The listing builds one solid part. Answer for the finished solid, in the listing's coordinates (mm). A direction names the side the tool comes from. Give positions to 0.01 mm unless a question says otherwise; leave off trailing zeros. Order: outer loops, then holes, each group sorted by start corner. A loop starts at its lowest first (then second) coordinate and runs counter-clockwise, first axis right, second up. Notation, with made-up numbers: (70.25, 67.5) - (93.25, 67.5) arc R31 ccw to (93.25, 106.5) - close; hole circle Ø4 at (-19, 72.5). An arc over 180 degrees is marked (long way). Use a Markdown table: item, result. Add a question column.
1) Flat-ended cylindrical pins translate along their axes: pin 1 (0.9 mm diameter, centred on x = 36, z = 3.5, fed in from +Y); pin 2 (3.5 mm diameter, centred on x = -31.5, z = 2.5, fed in from -Y); pin 3 (1.8 mm diameter, centred on x = 12.5, z = 2, fed in from -Y). Find the tip coordinate at first contact, or state that the pin passes through.
2) For faces 4 (the face through (-28.752, -19.875, 3.042)), 5 (the face through (11.39, -18.34, 2.96)), 6 (the face through (0, 11, 3)), 7 (the face through (38.483, 8.961, 3.042)), 8 (the face through (-8.11, 70.83, 3.04)), determine the directions among +Z, -Z, +X, -X, +Y, -Y from which every point of the face is accessible in a straight line to the end or side of a thin tool.
3) Find section B-B, the plane x = 13. Determine the outline of the cut face in (y, z), plus the area to 3 significant figures.
4) Find section C-C, the plane y = 47. Determine the outline of the cut face in (x, z).
5) Straight lines are drawn through the part: line 1 (X direction, y = 4.5, z = 0.4); line 2 (X direction, y = 11.5, z = 2.5); line 3 (X direction, y = 7.5, z = 0.85). For each, find the intervals that lie inside material, in ascending order.
6) Find section D-D, the plane x = -3.5. Determine the outline of the cut face in (y, z), plus the area to 3 significant figures.
7) The mould has two halves that part along X. Classify faces 1 (the face through (-28, 0, 3)), 2 (the face through (-18, 71.455, 3)), 3 (the face through (-27.851, 70.864, 3.042)): released by +X, released by -X, zero draft, split by the parting line, or undercut.
8) Find section A-A, the plane y = -11. Determine the outline of the cut face in (x, z).
from build123d import *

# Parameters (mm, degrees)
F1_DEPTH = 6
F2_R     = 2.5
F3_R     = 1.5


with BuildPart() as f1:
    # F0 (on Top) → F1 (new body)
    with BuildSketch(Plane.XY):
        with BuildLine():
            Line((30, 0), (0, 0))
            Line((0, 0), (0, 20))
            Line((0, 20), (-7.605883, 71.455397))
            Line((-7.605883, 71.455397), (-28.394117, 71.455397))
            Line((-28.394117, 71.455397), (-36, 20))
            Line((-36, 20), (-36, -20.588065))
            Line((-36, -20.588065), (-28, -20.588065))
            Line((-28, -20.588065), (-28, 19.411935))
            Line((-28, 19.411935), (-22, 60.003195))
            ThreePointArc((-22, 60.003195), (-18, 63.455397), (-14, 60.003195))
            Line((-14, 60.003195), (-8, 19.411935))
            Line((-8, 19.411935), (-8, -37))
            ThreePointArc((-8, -37), (-5.506746, -40.705363), (-1.135141, -39.79152))
            Line((-1.135141, -39.79152), (35.638156, -2.052121))
            Line((35.638156, -2.052121), (40.024769, 10))
            Line((40.024769, 10), (33.639702, 10))
            Line((33.639702, 10), (30, 0))
        make_face()
        Polygon((-1, -31.055363), (-1, -6), (23.413963, -6), align=None, mode=Mode.SUBTRACT)
    extrude(amount=F1_DEPTH)

    # F2
    f2_edges = [f1.edges().sort_by_distance(p)[0] for p in [
        (-36, 20, 3),
        (-28.394117, 71.455397, 3),
        (-7.605883, 71.455397, 3),
        (33.639702, 10, 3),
        (40.024769, 10, 3),
        (-8, 19.411935, 3),
        (0, 20, 3),
        (0, 0, 3),
        (30, 0, 3),
        (35.638156, -2.052121, 3),
        (-1, -6, 3),
        (-36, -20.588065, 3),
        (-28, -20.588065, 3),
        (-28, 19.411935, 3),
    ]]
    fillet(f2_edges, radius=F2_R)

    # F3
    f3_edges = [f1.edges().sort_by_distance(p)[0] for p in [
        (23.413963, -6, 3),
        (-1, -31.055363, 3),
    ]]
    fillet(f3_edges, radius=F3_R)


solid = f1.part
The answers:
| question | item | result |
|---|---|---|
| 1 | pin 1 | y = 10 |
| 1 | pin 2 | y = -20.59 |
| 1 | pin 3 | y = -26.72 |
| 2 | face 4 | +Z, -Z, -Y |
| 2 | face 5 | +Z, -Z |
| 2 | face 6 | +Z, -Z, +Y |
| 2 | face 7 | +Z, -Z, +X |
| 2 | face 8 | +Z, -Z, +X, +Y |
| 3 | outline | (-25.29, 0) - (-16.69, 0) - (-16.69, 6) - (-25.29, 6) - close; (-6, 0) - (0, 0) - (0, 6) - (-6, 6) - close |
| 3 | area | 87.6 mm2 |
| 4 | outline | (-32.01, 0) - (-23.92, 0) - (-23.92, 6) - (-32.01, 6) - close; (-12.08, 0) - (-3.99, 0) - (-3.99, 6) - (-12.08, 6) - close |
| 5 | line 1 | -36 to -28, -8 to 0, 31.64 to 38.02 |
| 5 | line 2 | -36 to -28, -8 to 0 |
| 5 | line 3 | -36 to -28, -8 to 0, 32.73 to 38.95 |
| 6 | outline | (-40.97, 0) - (43.68, 0) - (43.68, 6) - (-40.97, 6) - close |
| 6 | area | 508 mm2 |
| 7 | face 1 | undercut |
| 7 | face 2 | zero draft |
| 7 | face 3 | released by -X |
| 8 | outline | (-36, 0) - (-28, 0) - (-28, 6) - (-36, 6) - close; (-8, 0) - (-1, 0) - (-1, 6) - (-8, 6) - close; (18.54, 0) - (26.92, 0) - (26.92, 6) - (18.54, 6) - close |
